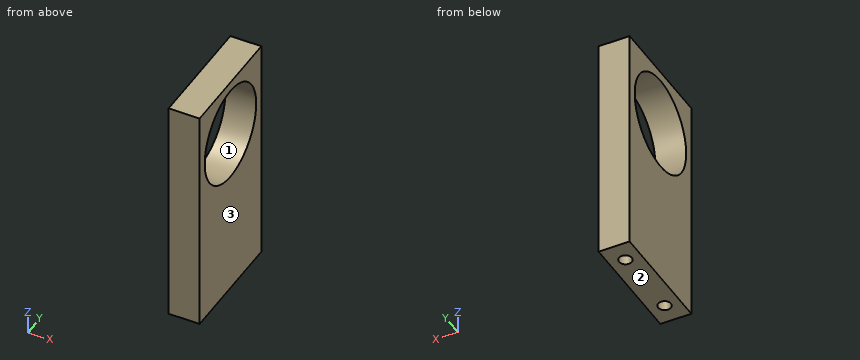
```python
from build123d import *

# Parameters (mm, degrees)
CYLINDER018_R     = 1.65
CYLINDER018_DEPTH = 20
CYLINDER019_R     = 1.65
CYLINDER019_DEPTH = 20
CYLINDER011_R     = 12.5
CYLINDER011_DEPTH = 10
BOX002_W          = 8
BOX002_H          = 30
BOX002_DEPTH      = 60


with BuildPart() as zylinder018:
    # Cylinder018 → Cylinder018 (new body)
    with BuildSketch(Plane(origin=(4, 38, 10), x_dir=(1, 0, 0), z_dir=(0, 0, 1))):
        Circle(CYLINDER018_R)
    extrude(amount=CYLINDER018_DEPTH)


with BuildPart() as compound003:
    # Cylinder019 → Cylinder019 (new body)
    with BuildSketch(Plane(origin=(4, 57, 10), x_dir=(1, 0, 0), z_dir=(0, 0, 1))):
        Circle(CYLINDER019_R)
    extrude(amount=CYLINDER019_DEPTH)

    # Compound003: union Zylinder018
    add(zylinder018.part)


with BuildPart() as zylinder011:
    # Cylinder011 → Cylinder011 (new body)
    with BuildSketch(Plane(origin=(0, 47.5, 60), x_dir=(0, 0, -1), z_dir=(1, 0, 0))):
        Circle(CYLINDER011_R)
    extrude(amount=CYLINDER011_DEPTH)


with BuildPart() as cameraholder:
    # Box002 → Box002 (new body)
    with BuildSketch(Plane(origin=(0, 32.5, 15), x_dir=(1, 0, 0), z_dir=(0, 0, 1))):
        with Locations((4, 15)):
            Rectangle(BOX002_W, BOX002_H)
    extrude(amount=BOX002_DEPTH)

    # Cut003: cut Zylinder011
    add(zylinder011.part, mode=Mode.SUBTRACT)

    # Cut007: cut Compound003
    add(compound003.part, mode=Mode.SUBTRACT)


solid = cameraholder.part
```
Input: part model. Units: mm. Frame: model coordinates. Face numbers are marked on the shaded views. Coordinates: 2 decimals unless noted, no trailing zeros. Write each loop counter-clockwise with the first axis right and the second up, starting at its lowest first coordinate (ties: lowest second). Pieces come first, ordered by that corner, then holes. Notation, with made-up numbers: (-10.75, 72) -> (30.25, 72) arc R32 ccw to (30.25, 98) -> close; hole circle Ø1 at (-22.75, 81). An arc over 180 degrees is marked (long way). Write each question's results on one line, items separated by ' | '.
Item 1: Section query D-D on y = 57. Return loops of the section in (x, z), plus the area to 3 significant figures.
Conclusion:
outline: (0, 15) -> (2.35, 15) -> (2.35, 30) -> (5.65, 30) -> (5.65, 15) -> (8, 15) -> (8, 51.88) -> (0, 51.88) -> close; (0, 68.12) -> (8, 68.12) -> (8, 75) -> (0, 75) -> close | area: 301 mm^2
Item 2: Material intervals for probe 1 along Y at (x, z) = (4, 23.75); probe 2 along Y at (x, z) = (2.5, 60); probe 3 along X at (y, z) = (57, 21), sorted ascending.
Conclusion:
probe 1: y = 32.5 to 36.35, 39.65 to 55.35, 58.65 to 62.5 | probe 2: y = 32.5 to 35, 60 to 62.5 | probe 3: x = 0 to 2.35, 5.65 to 8
Item 3: Section query C-C on x = 4. Return loops of the section in (y, z).
Conclusion:
outline: (32.5, 15) -> (36.35, 15) -> (36.35, 30) -> (39.65, 30) -> (39.65, 15) -> (55.35, 15) -> (55.35, 30) -> (58.65, 30) -> (58.65, 15) -> (62.5, 15) -> (62.5, 75) -> (32.5, 75) -> close; hole circle Ø25 at (47.5, 60)
Item 4: Pin query (flat end, axial travel): pin 1 Ø10 at (y, z) = (44, 67) entering from -X. Return the tip coordinate at first contact, or that it passes through.
Conclusion:
pin 1: stops at x = 0
Item 5: Mould query, pull axis Z, two halves, no side actions, for the marked faces 1, 2 and 3. Classes: +Z half, -Z half, draft (parallel to the pull), parting line (faces both ways), or undercut.
Conclusion:
face 1: undercut | face 2: -Z half | face 3: draft
Item 6: Section query B-B on z = 52.5. Return loops of the section in (x, y), plus the area to 3 significant figures.
Conclusion:
outline: (0, 32.5) -> (8, 32.5) -> (8, 37.5) -> (0, 37.5) -> close; (0, 57.5) -> (8, 57.5) -> (8, 62.5) -> (0, 62.5) -> close | area: 80.0 mm^2
Item 7: Section query A-A on y = 51. Return loops of the section in (x, z).
Conclusion:
outline: (0, 15) -> (8, 15) -> (8, 48) -> (0, 48) -> close; (0, 72) -> (8, 72) -> (8, 75) -> (0, 75) -> close
